Geometry check sheet. Reference: the model listing, model coordinates, mm. A direction names the side the tool comes from. Give positions to 0.01 mm unless a question says otherwise; leave off trailing zeros. Write each loop counter-clockwise with the first axis right and the second up, starting at its lowest first coordinate (ties: lowest second). Pieces come first, ordered by that corner, then holes. Notation, with made-up numbers: M -24,56.5 L 24,56.5 A16 cw 24,62.5 Z; hole C -2.75,43.25 d5. An arc over 180 degrees is marked long. Write each question's results on one line, items separated by ' | '.
```python
from build123d import *

# Parameters (mm, degrees)
SKETCH1_R           = 18
BOSS_EXTRUDE1_DEPTH = 10
BOSS_EXTRUDE2_DEPTH = 2
BOSS_EXTRUDE4_DEPTH = 20


with BuildPart() as part:
    # Sketch1 → Boss-Extrude1 (new body)
    with BuildSketch(Plane(origin=(0, 0, 0), x_dir=(0, 0, -1), z_dir=(1, 0, 0))):
        Circle(SKETCH1_R)
    extrude(amount=BOSS_EXTRUDE1_DEPTH)

    # Sketch2 → Boss-Extrude2 (add)
    with BuildSketch(Plane.ZY):
        with BuildLine():
            Line((-10, 14.966629547), (-10, 30))
            Line((-10, 30), (10, 30))
            Line((10, 30), (10, 14.966629547))
            ThreePointArc((10, 14.966629547), (0, -18), (-10, 14.966629547))
        make_face()
    extrude(amount=BOSS_EXTRUDE2_DEPTH)

    # Sketch5 → Boss-Extrude4 (add)
    with BuildSketch(Plane(origin=(0, 0, -10), x_dir=(-1, 0, 0), z_dir=(0, 0, -1))):
        Polygon((-2, 36), (-48, 36), (-48, 33), (-2, 33), (0, 30), (0, 14.966629547), (2, 14.966629547), (2, 30), align=None)
    extrude(amount=-BOSS_EXTRUDE4_DEPTH)


solid = part.part
```
Q1. Section check B-B (y = 0). Enter the section's corners in (x, z), then the cut area to 3 significant figures.
Answer key:
outline: M -2,-18 L 10,-18 L 10,18 L -2,18 Z | area: 432 mm2
Q2. Material ranges on probe 1 along Y at (x, z) = (39, -5); probe 2 along X at (y, z) = (20.5, 2); probe 3 along X at (y, z) = (-4, 6.5), recorded low to high. Write a range as [from, to].
Answer key:
probe 1: y = [33, 36] | probe 2: x = [-2, 0] | probe 3: x = [-2, 10]
Q3. Section check C-C (x = 13.5). Enter the section's corners in (y, z), then the cut area to 3 significant figures.
Answer key:
outline: M 33,-10 L 36,-10 L 36,10 L 33,10 Z | area: 60.0 mm2
Q4. Section check A-A (z = 0). Enter the section's corners in (x, y).
Answer key:
outline: M -2,-18 L 10,-18 L 10,18 L 0,18 L 0,30 L 2,33 L 48,33 L 48,36 L 2,36 L -2,30 Z
Q5. Access from +Z, -Z, +X, -X, +Y, -Y to the whole of each face (thin tool, end or side, straight path). Record for faces 4 (the face through (10, 0, 0)), 5 (the face through (19, 34, 10)), 6 (the face through (25, 33, 0)).
Answer key:
face 4: +Z, -Z, +X, -Y | face 5: +Z, +X, -X, +Y | face 6: +Z, -Z, +X
Q6. Depth check by flat-ended pin: P1, Ø12, axis at x = 24.5, z = 3, coming from the -Y side; P2, Ø3, axis at x = 5.5, z = 11, coming from the +Y side; P3, Ø16.5, axis at y = 19, z = 2, coming from the +X side. Enter the tip coordinate at first touch or a pass-through.
Answer key:
P1: stops at y = 33 | P2: stops at y = 36 | P3: stops at x = 10
Q7. Release check for a two-part mould opening along Y. For faces 1 (the face through (0, 24, 0)), 2 (the face through (0, 33, 0)), 3 (the face through (19, 34, -10)) record: released by +Y, released by -Y, zero draft, split by the parting line, or undercut.
Answer key:
face 1: undercut | face 2: released by +Y | face 3: zero draft
Q8. Section check D-D (y = 25.5). Enter the section's corners in (x, z), then the cut area to 3 significant figures.
Answer key:
outline: M -2,-10 L 0,-10 L 0,10 L -2,10 Z | area: 40.0 mm2
